Input: part model. Units: mm. Frame: model coordinates. A direction names the side the tool comes from. Give positions to 0.01 mm unless a question says otherwise; leave off trailing zeros. Loops run counter-clockwise (first coordinate to the right, second up) from the corner with the lowest first, then second, coordinate; pieces in that order, holes last. Notation, with made-up numbers: M 82,36.5 L 127,36.5 A33 cw 127,64.5 Z; hole C -25,42 d3. An arc over 180 degrees is marked long. One line per item, written item: value. Start each with the question number.
(1) Ray query, line 1 along Y through (x, z) = (0, 1.5); line 2 along Y through (x, z) = (-11, 37); line 3 along Z through (x, y) = (3, -8.5). Return the intervals inside material, ascending. Write a range as from..to.
(2) Section C-C on y = -5.25. Output: boundary loops of the cut face in (x, z).
(3) Section D-D on z = -3. Output: boundary loops of the cut face in (x, y), plus the area to 3 significant figures.
(4) Section A-A on y = 0. Output: boundary loops of the cut face in (x, z), plus the area to 3 significant figures.
(5) Pin query (flat end, axial travel): P1, Ø2, axis at x = 3, y = -4, coming from the -Z side; P2, Ø8, axis at x = -8.5, z = 4.5, coming from the -Y side; P3, Ø6, axis at x = -11, z = 32, coming from the -Y side. Return the tip coordinate at first contact, or that it passes through.
(6) Section B-B on z = 45.5. Output: boundary loops of the cut face in (x, y).
(7) Pull-direction query (Y, two-part tool) for faces 1 (the flat face through (3, -8, -6.528)), 2 (the flat face through (-3.675, -8.501, 37.922)), 3 (the flat face through (-5.438, -7.282, 37.922)); classes: released by +Y, released by -Y, zero draft, split by the parting line, or undercut.
(8) Access query for faces 4 (the flat face through (-7, 12, 25.4)), 5 (the cylindrical face through (-1.78, -8.01, 9.21)), 6 (the flat face through (-1.44, -2.53, 37.92)). Directions: +Z, -Z, +X, -X, +Y, -Y. A direction counts if a zero-diameter tool reaches every point of the face in a straight line with its end or side. Return the directions, or none.
```python
from build123d import *

# Parameters (mm, degrees)
F2_FACE_R   = 12.8778
F2_FACE_R_2 = 8.2042
F3_DEPTH    = 25.4
F4_W        = 12.40562
F4_H        = 2.135868
F5_DEPTH    = 25.4


with BuildPart() as f2:
    # F1 (on Front) → F2 (revolve)
    with BuildSketch(Plane.XZ):
        Polygon((12.8778, 0), (8.2042, 0), (8.2042, -6.5278), (10.50925, -6.5278), (10.50925, -1.7145), (12.8778, -1.7145), align=None)
    revolve(axis=Axis((0, 0, 18.280845), (0, 0, 1)))

    # F2_face (on face) → F3 (join)
    with BuildSketch(Plane.XY):
        Circle(F2_FACE_R)
        Circle(F2_FACE_R_2, mode=Mode.SUBTRACT)
    extrude(amount=F3_DEPTH)

    # F4 (on face) → F5 (join)
    with BuildSketch(Plane.XY.offset(25.4)):
        with Locations((9.112263, 0)):
            Rectangle(F4_W, F4_H)
        Polygon((6.732679, 13.797209), (0.529869, 3.053627), (2.379584, 1.985693), (8.582394, 12.729275), align=None)
        Polygon((-8.582394, 12.729275), (-2.379584, 1.985693), (-0.529869, 3.053627), (-6.732679, 13.797209), align=None)
        with Locations((-9.112263, 0)):
            Rectangle(F4_W, F4_H)
        Polygon((-6.732679, -13.797209), (-0.529869, -3.053627), (-2.379584, -1.985693), (-8.582394, -12.729275), align=None)
        Polygon((8.582394, -12.729275), (2.379584, -1.985693), (0.529869, -3.053627), (6.732679, -13.797209), align=None)
    extrude(amount=F5_DEPTH)


solid = f2.part
```
Output values:
1. line 1: y = -12.88..-8.2, 8.2..12.88
1. line 2: y = -1.07..1.07
1. line 3: z = -6.53..25.4
2. outline: M -11.76,-1.71 L -9.1,-1.71 L -9.1,-6.53 L -6.3,-6.53 L -6.3,25.4 L -11.76,25.4 Z; M -4.26,25.4 L -1.8,25.4 L -1.8,50.8 L -4.26,50.8 Z; M 1.8,25.4 L 4.26,25.4 L 4.26,50.8 L 1.8,50.8 Z; M 6.3,-6.53 L 9.1,-6.53 L 9.1,-1.71 L 11.76,-1.71 L 11.76,25.4 L 6.3,25.4 Z
3. outline: C 0,0 d21.02; hole C 0,0 d16.41
3. area: 136 mm²
4. outline: M -15.32,25.4 L -12.88,25.4 L -12.88,-1.71 L -10.51,-1.71 L -10.51,-6.53 L -8.2,-6.53 L -8.2,25.4 L -2.91,25.4 L -2.91,50.8 L -15.32,50.8 Z; M 2.91,25.4 L 8.2,25.4 L 8.2,-6.53 L 10.51,-6.53 L 10.51,-1.71 L 12.88,-1.71 L 12.88,25.4 L 15.32,25.4 L 15.32,50.8 L 2.91,50.8 Z
4. area: 906 mm²
5. P1: stops at z = 25.4
5. P2: stops at y = -12.07
5. P3: stops at y = -13.07
6. outline: M -15.32,-1.07 L -2.91,-1.07 L -2.91,1.07 L -15.32,1.07 Z; M -8.58,-12.73 L -6.73,-13.8 L -0.53,-3.05 L -2.38,-1.99 Z; M -8.58,12.73 L -2.38,1.99 L -0.53,3.05 L -6.73,13.8 Z; M 0.53,-3.05 L 6.73,-13.8 L 8.58,-12.73 L 2.38,-1.99 Z; M 0.53,3.05 L 2.38,1.99 L 8.58,12.73 L 6.73,13.8 Z; M 2.91,-1.07 L 15.32,-1.07 L 15.32,1.07 L 2.91,1.07 Z
7. face 1: zero draft
7. face 2: released by -Y
7. face 3: undercut
8. face 4: -Z, -X, +Y
8. face 5: -Z
8. face 6: +Z, -Z
